The listing builds one solid part. Answer for the finished solid, in the listing's coordinates (mm). A direction names the side the tool comes from. Give positions to 0.01 mm unless a question says otherwise; leave off trailing zeros. Write each loop counter-clockwise with the first axis right and the second up, starting at its lowest first coordinate (ties: lowest second). Pieces come first, ordered by that corner, then holes. Notation, with made-up numbers: M 32,-39 L 84,-39 A34 ccw 84,-4 Z; hole C -32.5,28 d9. An arc over 180 degrees is marked long. Return JSON: item names as keys, results as strings.
Autodesk Inventor part; units mm, degrees
ref_plane "YZ Plane" through (0, 0, 0) normal (1, 0, 0) x (0, 1, 0)
ref_plane "XZ Plane" through (0, 0, 0) normal (0, 1, 0) x (-1, 0, 0)
ref_plane "XY Plane" through (0, 0, 0) normal (0, 0, 1) x (1, 0, 0)
sketch "スケッチ1" plane through (0, 0, 0) normal (1, 0, 0) x (0, 1, 0)
  line L0 (0, 0) -> (15, 0)
  line L1 (15, 0) -> (15, -10)
  line L2 (15, -10) -> (0, -10)
  line L3 (0, -10) -> (0, 0)
  line L4 (1, -1) -> (14, -1)
  line L5 (14, -1) -> (14, -9)
  line L6 (14, -9) -> (1, -9)
  line L7 (1, -9) -> (1, -1)
  dimension "d0" = 15
  dimension "d1" = 10
  dimension "d2" = 13
  dimension "d3" = 8
  dimension "d4" = 1
  dimension "d5" = 1
extrude "押し出し1" add sketch "スケッチ1" along normal blind 106
sketch "スケッチ2" plane through (0, 15, 0) normal (0, 1, 0) x (1, 0, 0)
  line L0 (0, 9) -> (0, 1)
  line L1 (0, 5) -> (120, 5)
  line L2 (106, 10) -> (106, 0)
  point P0 (0, 0)
  point P1 (5, 5)
  point P2 (101, 5)
  point P3 (106, 0)
  dimension "d8" = 5
  dimension "d9" = 5
hole "穴1" at (5, 15, -5) at (101, 15, -5) direction (0, -1, 0) diameter 3.2 end through all
sketch "スケッチ3" plane through (0, 0, 0) normal (0, 0, 1) x (1, 0, 0)
  line L0 (0, 0) -> (0, 15)
  line L1 (0, 7.5) -> (106, 7.5)
  line L2 (106, 0) -> (106, 15)
  point P0 (23, 7.5)
  point P1 (83, 7.5)
  point P2 (53, 7.5)
  dimension "d17" = 30
  dimension "d18" = 30
hole "穴2" at (23, 7.5, 0) at (83, 7.5, 0) direction (0, 0, -1) diameter 3.2 end through all
properties part number "link2_pipe1" material "アルミニウム 6061"
Item 1: A cutting plane is placed at C-C, the plane x = 61.5. Write down the section's boundary in (y, z), plus the area to 3 significant figures.
Geometry results:
{"outline": "M 0,-10 L 15,-10 L 15,0 L 0,0 Z; hole M 1,-9 L 14,-9 L 14,-1 L 1,-1 Z", "area": "46.0 mm2"}
Item 2: Determine the mould class of faces 3 (the flat face through (52, 15, -5)), 4 (the cylindrical face through (21.414, 7.708, -0.507)), 5 (the cylindrical face through (4.93, 14.49, -6.6)) for opening direction Y: +Y half, -Y half, draft (parallel to the pull), parting line (faces both ways), or undercut.
Geometry results:
{"face 3": "+Y half", "face 4": "undercut", "face 5": "draft"}
Item 3: A cutting plane is placed at D-D, the plane x = 101. Write down the section's boundary in (y, z), plus the area to 3 significant figures.
Geometry results:
{"outline": "M 0,-10 L 15,-10 L 15,-6.6 L 14,-6.6 L 14,-9 L 1,-9 L 1,-6.6 L 0,-6.6 Z; M 0,-3.4 L 1,-3.4 L 1,-1 L 14,-1 L 14,-3.4 L 15,-3.4 L 15,0 L 0,0 Z", "area": "39.6 mm2"}
Item 4: A cutting plane is placed at B-B, the plane y = 7.5. Write down the section's boundary in (x, z).
Geometry results:
{"outline": "M 0,-10 L 21.4,-10 L 21.4,-9 L 0,-9 Z; M 0,-1 L 21.4,-1 L 21.4,0 L 0,0 Z; M 24.6,-10 L 81.4,-10 L 81.4,-9 L 24.6,-9 Z; M 24.6,-1 L 81.4,-1 L 81.4,0 L 24.6,0 Z; M 84.6,-10 L 106,-10 L 106,-9 L 84.6,-9 Z; M 84.6,-1 L 106,-1 L 106,0 L 84.6,0 Z"}
Item 5: A cutting plane is placed at A-A, the plane z = -5. Write down the section's boundary in (x, y), plus the area to 3 significant figures.
Geometry results:
{"outline": "M 0,0 L 3.4,0 L 3.4,1 L 0,1 Z; M 0,14 L 3.4,14 L 3.4,15 L 0,15 Z; M 6.6,0 L 99.4,0 L 99.4,1 L 6.6,1 Z; M 6.6,14 L 99.4,14 L 99.4,15 L 6.6,15 Z; M 102.6,0 L 106,0 L 106,1 L 102.6,1 Z; M 102.6,14 L 106,14 L 106,15 L 102.6,15 Z", "area": "199 mm2"}
Item 6: Find the intervals of material crossed by line 1 (X direction, y = 7.5, z = -9.6); line 2 (X direction, y = 14.3, z = -5); line 3 (Z direction, x = 52, y = 10), in increasing order.
Geometry results:
{"line 1": "x = 0 to 21.4, 24.6 to 81.4, 84.6 to 106", "line 2": "x = 0 to 3.4, 6.6 to 99.4, 102.6 to 106", "line 3": "z = -10 to -9, -1 to 0"}
Item 7: Which of the six approach directions +Z, -Z, +X, -X, +Y, -Y give full straight-line access (tool end or side, diameter ignored) to faces 1 (the cylindrical face through (81.414, 7.708, -0.507)), 2 (the flat face through (52, 1, -5))?
Geometry results:
{"face 1": "+Z, -Z", "face 2": "+X, -X"}
